Check sheet for the modelled part. Datum: model origin and axes. Units: mm. Face numbers are marked on the shaded views. A direction names the side the tool comes from. Give positions to 0.01 mm unless a question says otherwise; leave off trailing zeros. Loops run counter-clockwise (first coordinate to the right, second up) from the corner with the lowest first, then second, coordinate; pieces in that order, holes last. Notation, with made-up numbers: (57.5, 68.25) -> (74.5, 68.25) arc R18 ccw to (74.5, 93.25) -> close; hole circle Ø3 at (71.5, 22). An arc over 180 degrees is marked (long way). Answer as CSV lines item,"result". Start each with the question number.
(1) Access from +Z, -Z, +X, -X, +Y, -Y to the whole of each face (thin tool, end or side, straight path). Record for the marked faces 4 and 5.
(2) Section check B-B on x = 0. State how many separate pieces and enclosed holes the cut face has, plus the area to 3 significant figures.
(3) Section check C-C on y = -8. Enter the section's corners in (x, z).
(4) Gauge pin test, flat ends, axial feed: pin 1 Ø1.8 at (x, y) = (13, 3.5) entering from +Z; pin 2 Ø1.1 at (x, y) = (-13.5, 3.5) entering from -Z; pin 3 Ø2.5 at (x, y) = (-5.5, 3.5) entering from -Z. Record the tip position at first contact, or that the pin passes through.
(5) Release check for a two-part mould opening along X. For the marked faces 1, 2 and 3 record: pulls with the +X half, pulls with the -X half, needs draft (parallel to the pull), parting line crosses it, or undercut.
(6) Section check A-A on z = 0. Enter the section's corners in (x, y), plus the area to 3 significant figures.
(7) Material ranges on line 1 (Y direction, x = 25.5, z = 15); line 2 (X direction, y = -35.5, z = -17); line 3 (Z direction, x = 12, y = -21.5), recorded low to high. Write a range as from..to.
(8) Section check D-D on y = -3. Enter the section's corners in (x, z), plus the area to 3 significant figures.
Autodesk Inventor part; units mm, degrees
ref_plane "YZ Plane" through (0, 0, 0) normal (1, 0, 0) x (0, 1, 0)
ref_plane "XZ Plane" through (0, 0, 0) normal (0, 1, 0) x (-1, 0, 0)
ref_plane "XY Plane" through (0, 0, 0) normal (0, 0, 1) x (1, 0, 0)
sketch "Skizze1" plane through (0, 0, 0) normal (0, 0, 1) x (1, 0, 0)
  line L0 (-25, -40) -> (-25, 0)
  line L1 (-25, 0) -> (-31.75, 0)
  line L2 (-31.75, 0) -> (-31.75, 5)
  line L3 (-31.75, 5) -> (-15, 5)
  line L4 (-22, -40) -> (-22, -4.0415)
  line L5 (-22, -4.0415) -> (-15, 0)
  line L6 (-15, 0) -> (-15, 5)
  line L7 (-38.1, 0) -> (6.35, 0) construction
  line L8 (-22, -40) -> (-25, -40)
  line L9 (0, -49) -> (0, 14)
  point P0 (0, 0)
  dimension "d2" = 60
  dimension "d3" = 3
  dimension "d4" = 5
  dimension "d5" = 7
  dimension "d6" = 50
  dimension "d7" = 40
  dimension "d8" = 63.5
  dimension "d38" = 5
  dimension "d47" = 30
revolve "Umdrehung1" add sketch "Skizze1" angle 360 about axis through (0, -10, 0) along (0, 1, 0)
sketch "Skizze2" plane through (0, 5, 0) normal (0, 1, 0) x (1, 0, 0)
  circle A0 centre (0, 0) radius 15
  circle A1 centre (0, 0) radius 31.75
  line L0 (-44.45, 0) -> (44.45, 0) construction
  line L1 (0, 44.45) -> (0, -44.45) construction
  circle A2 centre (0, 0) radius 9.5
  circle A3 centre (0, 0) radius 11.5
  circle A4 centre (0, 0) radius 4
  circle A5 centre (0, 0) radius 3
  line L2 (-14.9666, 1) -> (-3.873, 1)
  line L3 (-3.873, -1) -> (-14.9666, -1)
  arc A6 (-3.873, 1) -> (-3.873, -1) centre (0, 0) ccw
  arc A7 (-14.9666, 1) -> (-14.9666, -1) centre (0, 0) ccw
  line L4 (-8.3493, -12.4615) -> (-2.8025, -2.8541)
  line L5 (-1.0705, -3.8541) -> (-6.6173, -13.4615)
  arc A8 (-8.3493, -12.4615) -> (-6.6173, -13.4615) centre (0, 0) ccw
  arc A9 (-2.8025, -2.8541) -> (-1.0705, -3.8541) centre (0, 0) ccw
  line L6 (6.6173, -13.4615) -> (1.0705, -3.8541)
  line L7 (2.8025, -2.8541) -> (8.3493, -12.4615)
  arc A10 (6.6173, -13.4615) -> (8.3493, -12.4615) centre (0, 0) ccw
  arc A11 (1.0705, -3.8541) -> (2.8025, -2.8541) centre (0, 0) ccw
  line L8 (14.9666, -1) -> (3.873, -1)
  line L9 (3.873, 1) -> (14.9666, 1)
  arc A12 (14.9666, -1) -> (14.9666, 1) centre (0, 0) ccw
  arc A13 (3.873, -1) -> (3.873, 1) centre (0, 0) ccw
  line L10 (8.3493, 12.4615) -> (2.8025, 2.8541)
  line L11 (1.0705, 3.8541) -> (6.6173, 13.4615)
  arc A14 (8.3493, 12.4615) -> (6.6173, 13.4615) centre (0, 0) ccw
  arc A15 (2.8025, 2.8541) -> (1.0705, 3.8541) centre (0, 0) ccw
  line L12 (-6.6173, 13.4615) -> (-1.0705, 3.8541)
  line L13 (-2.8025, 2.8541) -> (-8.3493, 12.4615)
  arc A16 (-6.6173, 13.4615) -> (-8.3493, 12.4615) centre (0, 0) ccw
  arc A17 (-1.0705, 3.8541) -> (-2.8025, 2.8541) centre (0, 0) ccw
  dimension "d25" = 19
  dimension "d26" = 23
  dimension "d28" = 8
  dimension "d29" = 6
  dimension "d30" = 2
  dimension "d41" = 360
extrude "Extrusion1" add sketch "Skizze2" against normal blind 5 contours A0 L8 A3 L9 | L10 A3 L11 A0 | L9 A2 L10 A3 | A3 L8 A2 L9 | A0 L6 A3 L7 | A3 L7 A2 L8 | L10 A2 L11 A3 | A2 L8 A4 L9 | A3 L6 A2 L7 | L12 A3 L13 A0 | L11 A2 L12 A3 | L10 A4 L11 A2 | A4 | A0 L4 A3 L5 | A3 L5 A2 L6 | A2 L6 A4 L7 | L12 A2 L13 A3 | A3 L4 A2 L5 | L2 A3 L3 A0 | L13 A2 L2 A3 | L12 A4 L13 A2 | A3 L3 A2 L4 | A2 L4 A4 L5 | L2 A2 L3 A3 | L2 A4 L3 A2
chamfer "Fase1" distance 1 angle 45 2 edges at (31.75, 0, 0) (25, -40, 0)
sketch "Skizze3" plane through (0, 0, 0) normal (0, -1, 0) x (1, 0, 0)
  circle A0 centre (0, 0) radius 22
  arc A1 (-6.6173, -13.4615) -> (6.6173, -13.4615) centre (0, 0) ccw
  line L0 (6.6173, -13.4615) -> (4.8622, -10.4216)
  arc A2 (-4.8622, -10.4216) -> (4.8622, -10.4216) centre (0, 0) ccw
  line L1 (-4.8622, -10.4216) -> (-6.6173, -13.4615)
  line L2 (-8.3493, -12.4615) -> (-6.5942, -9.4216)
  arc A3 (-11.4564, -1) -> (-6.5942, -9.4216) centre (0, 0) ccw
  line L3 (-11.4564, -1) -> (-14.9666, -1)
  arc A4 (-14.9666, -1) -> (-8.3493, -12.4615) centre (0, 0) ccw
  line L4 (-14.9666, 1) -> (-11.4564, 1)
  arc A5 (-6.5942, 9.4216) -> (-11.4564, 1) centre (0, 0) ccw
  line L5 (-6.5942, 9.4216) -> (-8.3493, 12.4615)
  arc A6 (-8.3493, 12.4615) -> (-14.9666, 1) centre (0, 0) ccw
  line L6 (-6.6173, 13.4615) -> (-4.8622, 10.4216)
  arc A7 (4.8622, 10.4216) -> (-4.8622, 10.4216) centre (0, 0) ccw
  line L7 (4.8622, 10.4216) -> (6.6173, 13.4615)
  arc A8 (6.6173, 13.4615) -> (-6.6173, 13.4615) centre (0, 0) ccw
  line L8 (8.3493, 12.4615) -> (6.5942, 9.4216)
  arc A9 (11.4564, 1) -> (6.5942, 9.4216) centre (0, 0) ccw
  line L9 (11.4564, 1) -> (14.9666, 1)
  arc A10 (14.9666, 1) -> (8.3493, 12.4615) centre (0, 0) ccw
  arc A11 (3.8576, 8.6815) -> (-3.8576, 8.6815) centre (0, 0) ccw
  line L10 (-3.8576, 8.6815) -> (-1.0705, 3.8541)
  arc A12 (1.0705, 3.8541) -> (-1.0705, 3.8541) centre (0, 0) ccw
  line L11 (1.0705, 3.8541) -> (3.8576, 8.6815)
  line L12 (9.4472, -1) -> (3.873, -1)
  arc A13 (2.8025, -2.8541) -> (3.873, -1) centre (0, 0) ccw
  line L13 (2.8025, -2.8541) -> (5.5896, -7.6815)
  arc A14 (5.5896, -7.6815) -> (9.4472, -1) centre (0, 0) ccw
  circle A15 centre (0, 0) radius 3
  line L14 (3.8576, -8.6815) -> (1.0705, -3.8541)
  arc A16 (-1.0705, -3.8541) -> (1.0705, -3.8541) centre (0, 0) ccw
  line L15 (-1.0705, -3.8541) -> (-3.8576, -8.6815)
  arc A17 (-3.8576, -8.6815) -> (3.8576, -8.6815) centre (0, 0) ccw
  line L16 (5.5896, 7.6815) -> (2.8025, 2.8541)
  arc A18 (3.873, 1) -> (2.8025, 2.8541) centre (0, 0) ccw
  line L17 (3.873, 1) -> (9.4472, 1)
  arc A19 (9.4472, 1) -> (5.5896, 7.6815) centre (0, 0) ccw
  arc A20 (-5.5896, 7.6815) -> (-9.4472, 1) centre (0, 0) ccw
  line L18 (-9.4472, 1) -> (-3.873, 1)
  arc A21 (-2.8025, 2.8541) -> (-3.873, 1) centre (0, 0) ccw
  line L19 (-2.8025, 2.8541) -> (-5.5896, 7.6815)
  arc A22 (-9.4472, -1) -> (-5.5896, -7.6815) centre (0, 0) ccw
  line L20 (-5.5896, -7.6815) -> (-2.8025, -2.8541)
  arc A23 (-3.873, -1) -> (-2.8025, -2.8541) centre (0, 0) ccw
  line L21 (-3.873, -1) -> (-9.4472, -1)
  line L22 (14.9666, -1) -> (11.4564, -1)
  arc A24 (6.5942, -9.4216) -> (11.4564, -1) centre (0, 0) ccw
  line L23 (6.5942, -9.4216) -> (8.3493, -12.4615)
  arc A25 (8.3493, -12.4615) -> (14.9666, -1) centre (0, 0) ccw
  circle A26 centre (0, 0) radius 31.75
  line L24 (21.9773, -1) -> (17.9722, -1)
  line L25 (21.9773, 1) -> (17.9722, 1)
  arc A27 (17.9722, -1) -> (17.9722, 1) centre (0, 0) ccw
  arc A28 (21.9773, -1) -> (21.9773, 1) centre (0, 0) ccw
  arc A29 (9.8521, 15.0644) -> (8.1201, 16.0644) centre (0, 0) ccw
  line L26 (11.8547, 18.5329) -> (9.8521, 15.0644)
  arc A30 (11.8547, 18.5329) -> (10.1226, 19.5329) centre (0, 0) ccw
  line L27 (10.1226, 19.5329) -> (8.1201, 16.0644)
  arc A31 (-8.1201, 16.0644) -> (-9.8521, 15.0644) centre (0, 0) ccw
  line L28 (-10.1226, 19.5329) -> (-8.1201, 16.0644)
  arc A32 (-10.1226, 19.5329) -> (-11.8547, 18.5329) centre (0, 0) ccw
  line L29 (-11.8547, 18.5329) -> (-9.8521, 15.0644)
  arc A33 (-17.9722, 1) -> (-17.9722, -1) centre (0, 0) ccw
  line L30 (-21.9773, 1) -> (-17.9722, 1)
  arc A34 (-21.9773, 1) -> (-21.9773, -1) centre (0, 0) ccw
  line L31 (-21.9773, -1) -> (-17.9722, -1)
  arc A35 (-9.8521, -15.0644) -> (-8.1201, -16.0644) centre (0, 0) ccw
  line L32 (-11.8547, -18.5329) -> (-9.8521, -15.0644)
  arc A36 (-11.8547, -18.5329) -> (-10.1226, -19.5329) centre (0, 0) ccw
  line L33 (-10.1226, -19.5329) -> (-8.1201, -16.0644)
  arc A37 (8.1201, -16.0644) -> (9.8521, -15.0644) centre (0, 0) ccw
  line L34 (10.1226, -19.5329) -> (8.1201, -16.0644)
  arc A38 (10.1226, -19.5329) -> (11.8547, -18.5329) centre (0, 0) ccw
  line L35 (11.8547, -18.5329) -> (9.8521, -15.0644)
  dimension "d51" = 18
  dimension "d56" = 360
extrude "Extrusion5" add sketch "Skizze3" along normal up to surface (40 mm away) contours A0 L24 A27 L25 | L26 A29 L27 A0 | A0 L34 A37 L35 | L28 A31 L29 A0 | A0 L32 A35 L33 | L30 A33 L31 A0
properties part number "Unterdruckventil_Basis"
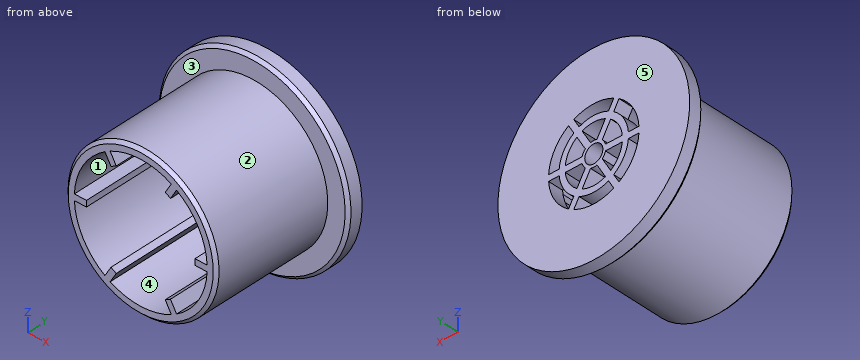
Working result:
1,face 4,"-Y"
1,face 5,"+Z, -Z, +X, -X, +Y"
2,separate pieces,"6"
2,enclosed holes,"0"
2,area,"464 mm^2"
3,outline,"circle Ø50 at (0, 0); hole (-21.98, -1) arc R22 ccw to (-11.85, -18.53) -> (-9.85, -15.06) arc R18.01 ccw to (-8.12, -16.06) -> (-10.12, -19.53) arc R22 ccw to (10.12, -19.53) -> (8.12, -16.06) arc R17.99 ccw to (9.85, -15.06) -> (11.85, -18.53) arc R22 ccw to (21.98, -1) -> (17.97, -1) arc R18 ccw to (17.97, 1) -> (21.98, 1) arc R22 ccw to (11.85, 18.53) -> (9.85, 15.06) arc R18.01 ccw to (8.12, 16.06) -> (10.12, 19.53) arc R22 ccw to (-10.12, 19.53) -> (-8.12, 16.06) arc R17.99 ccw to (-9.85, 15.06) -> (-11.85, 18.53) arc R22 ccw to (-21.98, 1) -> (-17.97, 1) arc R18 ccw to (-17.97, -1) -> close"
4,pin 1,"stops at z = 29.35"
4,pin 2,"stops at z = -28.99"
4,pin 3,"stops at z = -31.46"
5,face 1,"undercut"
5,face 2,"parting line crosses it"
5,face 3,"needs draft"
6,outline,"(-31.75, 1) -> (-30.75, 0) -> (-25, 0) -> (-25, -39) -> (-24, -40) -> (-18, -40) -> (-18, -1.73) -> (-15, 0) -> (-3, 0) -> (-3, 5) -> (-31.75, 5) -> close; (3, 0) -> (15, 0) -> (18, -1.73) -> (18, -40) -> (24, -40) -> (25, -39) -> (25, 0) -> (30.75, 0) -> (31.75, 1) -> (31.75, 5) -> (3, 5) -> close"
6,area,"851 mm^2"
7,line 1,"y = 0..5"
7,line 2,"x = -18.33..-13.96, -10.97..-8.66, 8.66..10.97, 13.96..18.33"
7,line 3,"z = -21.93..-18.44, 18.44..21.93"
8,outline,"circle Ø50 at (0, 0); hole (-20.17, -1) arc R20.2 ccw to (-10.95, -16.97) -> (-9.85, -15.06) arc R18.01 ccw to (-8.12, -16.06) -> (-9.22, -17.97) arc R20.2 ccw to (9.22, -17.97) -> (8.12, -16.06) arc R17.99 ccw to (9.85, -15.06) -> (10.95, -16.97) arc R20.2 ccw to (20.17, -1) -> (17.97, -1) arc R18 ccw to (17.97, 1) -> (20.17, 1) arc R20.2 ccw to (10.95, 16.97) -> (9.85, 15.06) arc R18.01 ccw to (8.12, 16.06) -> (9.22, 17.97) arc R20.2 ccw to (-9.22, 17.97) -> (-8.12, 16.06) arc R17.99 ccw to (-9.85, 15.06) -> (-10.95, 16.97) arc R20.2 ccw to (-20.17, 1) -> (-17.97, 1) arc R18 ccw to (-17.97, -1) -> close"
8,area,"708 mm^2"
